The listing builds one solid part. Answer for the finished solid, in the listing's coordinates (mm). Give positions to 0.01 mm unless a question says otherwise; leave off trailing zeros. Write each loop counter-clockwise with the first axis right and the second up, starting at its lowest first coordinate (ties: lowest second). Pieces come first, ordered by that corner, then holes. Notation, with made-up numbers: (87, 39) -> (99, 39) arc R24 ccw to (99, 52) -> close; hole circle Ø8 at (39, 8.5). An arc over 180 degrees is marked (long way). Use CSV: the item, a comma, the result in double quotes. Start each with the question number.
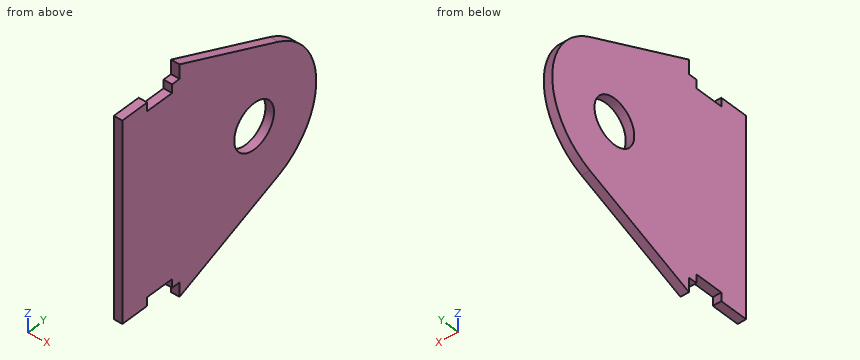
Autodesk Inventor part; units mm, degrees
ref_plane "YZ Plane" through (0, 0, 0) normal (1, 0, 0) x (0, 1, 0)
ref_plane "XZ Plane" through (0, 0, 0) normal (0, 1, 0) x (-1, 0, 0)
ref_plane "XY Plane" through (0, 0, 0) normal (0, 0, 1) x (1, 0, 0)
sketch "Sketch1" plane through (0, 0, 0) normal (1, 0, 0) x (0, 1, 0)
  circle A0 centre (0, 0) radius 8
  arc A1 (-25, 0) -> (9.8205, -22.9904) centre (0, 0) ccw construction
  line L0 (0, 0) -> (-30, 0) construction
  line L1 (-30, 0) -> (-30, -35) construction
  line L2 (-30, -40) -> (9.8205, -22.9904)
  line L3 (-30, 0) -> (-30, 35) construction
  line L4 (-30, 40) -> (9.8205, 22.9904)
  line L5 (-30, 0) -> (-33, 0) construction
  line L6 (-33, 0) -> (-33, -35) construction
  line L7 (-33, -35) -> (-30, -35)
  line L8 (-33, 0) -> (-33, 32) construction
  line L9 (-33, 35) -> (-30, 35)
  line L10 (-33, 35) -> (-43, 35) construction
  line L11 (-43, 35) -> (-43, -32) construction
  line L12 (-43, -35) -> (-33, -35) construction
  line L13 (-33, -35) -> (-33, -32)
  line L14 (-33, 35) -> (-43, 35) construction
  line L15 (-43, 35) -> (-43, 32)
  line L16 (-43, 32) -> (-33, 32)
  line L17 (-33, 32) -> (-33, 35)
  line L18 (-43, -35) -> (-33, -35) construction
  line L19 (-33, -35) -> (-33, -32)
  line L20 (-33, -32) -> (-43, -32)
  line L21 (-43, -32) -> (-43, -35)
  line L22 (-43, 35) -> (-46, 35)
  line L23 (-46, 35) -> (-46, -35) construction
  line L24 (-46, -35) -> (-43, -35)
  line L25 (-43, -35) -> (-43, -32)
  arc A2 (9.8205, 22.9904) -> (-25, 0) centre (0, 0) ccw construction
  arc A3 (9.8205, -22.9904) -> (9.8205, 22.9904) centre (0, 0) ccw
  line L26 (-30, 35) -> (-30, 40)
  line L27 (-30, -35) -> (-30, -40)
  line L28 (-33, 32) -> (-33, 35)
  line L29 (-33, -32) -> (-33, 35) construction
  line L30 (-43, -32) -> (-43, -35)
  line L31 (-43, 32) -> (-43, 35)
  line L32 (-43, -32) -> (-43, 32) construction
  line L33 (-46, 35) -> (-53, 35)
  line L34 (-53, 35) -> (-53, -35)
  line L35 (-53, -35) -> (-46, -35)
  point P0 (-43, -25)
  dimension "d0" = 16
  dimension "d1" = 50
  dimension "d2" = 30
  dimension "d4" = 40
  dimension "d5" = 40
  dimension "d8" = 3
  dimension "d19" = 10
  dimension "d20" = 70
  dimension "d21" = 3
  dimension "d22" = 3
  dimension "d23" = 3
  dimension "d24" = 35
  dimension "d25" = 7
  dimension "d26" = 70
  dimension "d27" = 7
extrude "Extrusion1" add sketch "Sketch1" along normal blind 3
properties part number "baseSoporte2" material "PMMA Plastic"
Q1. Section D-D on y = -32 is taken. Give the vertices of the cut face in (x, z), then the cut area to 3 significant figures.
Q2. Flat-ended cylindrical pins translate along their axes: pin 1 Ø1.5 at (x, z) = (1.5, -33.5) entering from +Y; pin 2 Ø1.5 at (x, z) = (1, 33) entering from +Y; pin 3 Ø1.5 at (x, y) = (1.5, -32) entering from -Z. Find the tip coordinate at first contact, or state that the pin passes through.
Q3. Section C-C on x = 1.6 is taken. Give the vertices of the cut face in (y, z).
Q4. Straight lines are drawn through the part: L1, parallel to Z at x = 1.95, y = -5 (3 decimals); L2, parallel to Z at x = 1.05, y = 0; L3, parallel to Z at x = 1.1, y = -32. For each, find the intervals that lie inside material, in ascending order.
Q5. Section A-A on z = 0 is taken. Give the vertices of the cut face in (x, y).
Q6. Section B-B on y = -5 is taken. Give the vertices of the cut face in (x, z) (3 decimals).
Output:
1,outline,"(0, -35) -> (3, -35) -> (3, 35) -> (0, 35) -> close"
1,area,"210 mm²"
2,pin 1,"y = -13.03"
2,pin 2,"y = -11.86"
2,pin 3,"z = -35"
3,outline,"(-53, -35) -> (-43, -35) -> (-43, -32) -> (-33, -32) -> (-33, -35) -> (-30, -35) -> (-30, -40) -> (9.82, -22.99) arc R25 ccw to (9.82, 22.99) -> (-30, 40) -> (-30, 35) -> (-33, 35) -> (-33, 32) -> (-43, 32) -> (-43, 35) -> (-53, 35) -> close; hole circle Ø16 at (0, 0)"
4,L1,"-29.321 to -6.245, 6.245 to 29.321"
4,L2,"-27.19 to -8, 8 to 27.19"
4,L3,"-35 to 35"
5,outline,"(0, -53) -> (3, -53) -> (3, -8) -> (0, -8) -> close; (0, 8) -> (3, 8) -> (3, 25) -> (0, 25) -> close"
6,outline,"(0, -29.321) -> (3, -29.321) -> (3, -6.245) -> (0, -6.245) -> close; (0, 6.245) -> (3, 6.245) -> (3, 29.321) -> (0, 29.321) -> close"
